```python
from build123d import *

# Parameters (mm, degrees)
BOSS_EXTRUDE1_DEPTH                    = 95
BOSS_EXTRUDE1_DEPTH_BACK               = 105
SKETCH1_R                              = 25
SKETCH2_R                              = 18
BOSS_EXTRUDE2_DEPTH                    = 46
CUT_EXTRUDE1_DEPTH                     = 10
CHAMFER1_SIZE                          = 0.5
SKETCH9_R                              = 10
CUT_EXTRUDE2_DEPTH                     = 30
CUT_EXTRUDE2_DRAFT                     = -8
SKETCH10_R                             = 6.5
CUT_EXTRUDE3_DEPTH                     = 50
SKETCH11_R                             = 6
CUT_EXTRUDE4_DEPTH                     = 249.527664456
CIRPATTERN1_COUNT                      = 4
CUT_EXTRUDE6_START                     = 69
SKETCH21_R                             = 25
SKETCH21_R_2                           = 20
CUT_EXTRUDE6_DEPTH                     = 27
CUT_EXTRUDE7_START                     = -105
SKETCH21_2_R                           = 25
SKETCH21_2_R_2                         = 20
CUT_EXTRUDE7_DEPTH                     = 39
CUT_EXTRUDE8_START                     = -162
SKETCH23_R                             = 25
SKETCH23_R_2                           = 23.75
CUT_EXTRUDE8_DEPTH                     = 135
SKETCH24_R                             = 20
SKETCH24_R_2                           = 19
CUT_EXTRUDE9_DEPTH                     = 20.1
M2_5X0_45_TAPPED_HOLE2_D               = 2.05
M2_5X0_45_TAPPED_HOLE2_DEPTH           = 5
M2_5X0_45_TAPPED_HOLE2_TIP             = 0.615882135
M2_5X0_45_TAPPED_HOLE2_ON_FACE_2_D     = 2.05
M2_5X0_45_TAPPED_HOLE2_ON_FACE_2_DEPTH = 5
M2_5X0_45_TAPPED_HOLE2_ON_FACE_2_TIP   = 0.615882135
CUT_EXTRUDE10_START                    = -12.1
SKETCH25_R                             = 20
SKETCH25_R_2                           = 19
CUT_EXTRUDE10_DEPTH                    = 12.1


with BuildPart() as part:
    # Sketch1 → Boss-Extrude1 (new, two sides: drawn at the far end of the back side and taken through both)
    with BuildSketch(Plane(origin=(0, 0, 0), x_dir=(1, 0, 0), z_dir=(0, 1, 0)).offset(-BOSS_EXTRUDE1_DEPTH_BACK)):
        with Locations(Location((0, 0, 0), (0, 0, 270))):
            Circle(SKETCH1_R)
    extrude(amount=BOSS_EXTRUDE1_DEPTH + BOSS_EXTRUDE1_DEPTH_BACK)

    # Sketch2 → Boss-Extrude2 (add)
    with BuildSketch(Plane(origin=(0, 95, 0), x_dir=(1, 0, 0), z_dir=(0, 1, 0))):
        with Locations(Location((0, 0, 0), (0, 0, 270))):
            Circle(SKETCH2_R)
    extrude(amount=BOSS_EXTRUDE2_DEPTH)

    # Sketch8 → Cut-Extrude1 (cut)
    with BuildSketch(Plane.XY.offset(-15)):
        with BuildLine():
            Line((3, 122), (3, 103))
            ThreePointArc((3, 103), (0, 100), (-3, 103))
            Line((-3, 103), (-3, 122))
            ThreePointArc((-3, 122), (0, 125), (3, 122))
        make_face()
    extrude(amount=-CUT_EXTRUDE1_DEPTH, mode=Mode.SUBTRACT)

    # Chamfer1
    chamfer1_edges = [part.edges().sort_by_distance(p)[0] for p in [
        (0, 141, -18),
    ]]
    chamfer(chamfer1_edges, length=CHAMFER1_SIZE)


with BuildPart() as cut_extrude2_tool:
    # Sketch9 → Cut-Extrude2 (with draft: the straight prism first)
    with BuildSketch(Plane.XZ.offset(105)):
        Circle(SKETCH9_R)
    extrude(amount=-CUT_EXTRUDE2_DEPTH)
    # Cut-Extrude2: the draft: its side faces are tilted about the plane it starts from
    cut_extrude2_sides = [cut_extrude2_tool.faces().sort_by_distance(p)[0] for p in [
        (-10, -90, 0),
    ]]
    draft(cut_extrude2_sides, Plane.XZ.offset(105), CUT_EXTRUDE2_DRAFT)


with BuildPart() as part_1:
    add(part.part)

    # Cut-Extrude2: cut by cut_extrude2_tool
    add(cut_extrude2_tool.part, mode=Mode.SUBTRACT)

    # Sketch10 → Cut-Extrude3 (cut)
    with BuildSketch(Plane.XZ.offset(105)):
        with Locations(Location((0, 0, 0), (0, 0, 270))):
            Circle(SKETCH10_R)
    extrude(amount=-CUT_EXTRUDE3_DEPTH, mode=Mode.SUBTRACT)

    # Sketch11 → Cut-Extrude4 (cut, through all)
    with BuildSketch(Plane(origin=(0, 141, 0), x_dir=(1, 0, 0), z_dir=(0, 1, 0))):
        with Locations(Location((0, 0, 0), (0, 0, 270))):
            Circle(SKETCH11_R)
    extrude(amount=-CUT_EXTRUDE4_DEPTH, mode=Mode.SUBTRACT)

    # Sketch15 → M5x0.8 Tapped Hole1 (revolve, cut)
    with BuildSketch(Plane(origin=(0, 141, -13), x_dir=(0, 0, 1), z_dir=(1, 0, 0))):
        Polygon((0, 0), (0, 12), (2.1, 10.7381927), (2.1, 0), align=None)
    m5x0_8_tapped_hole1 = revolve(axis=Axis((0, 147.35, -13), (0, -1, 0)), mode=Mode.SUBTRACT)

    # CirPattern1: M5x0.8 Tapped Hole1 ×4 about axis
    cirpattern1_axis = Axis((0, 0, 0), (0, 1, 0))
    for i in range(1, CIRPATTERN1_COUNT):
        add(m5x0_8_tapped_hole1.rotate(cirpattern1_axis, i * 360 / CIRPATTERN1_COUNT), mode=Mode.SUBTRACT)

    # Sketch20 → M2.5x0.45 Tapped Hole1 (revolve, cut)
    with BuildSketch(Plane(origin=(12.2, -105, 0), x_dir=(0, 0, -1), z_dir=(1, 0, 0))):
        Polygon((0, 0), (0, 9.35), (1.025, 8.734117865), (1.025, 0), align=None)
    m2_5x0_45_tapped_hole1 = revolve(axis=Axis((12.2, -111.35, 0), (0, 1, 0)), mode=Mode.SUBTRACT)

    # Mirror2: M2.5x0.45 Tapped Hole1 across plane
    add(m2_5x0_45_tapped_hole1.mirror(Plane(origin=(0, 0, 0), x_dir=(0, 0, 1), z_dir=(1, 0, 0))), mode=Mode.SUBTRACT)

    # Sketch21 → Cut-Extrude6 (cut)
    with BuildSketch(Plane(origin=(0, -1, 0), x_dir=(1, 0, 0), z_dir=(0, 1, 0)).offset(CUT_EXTRUDE6_START)):
        with Locations(Location((0, 0, 0), (0, 0, 270))):
            Circle(SKETCH21_R)
        with Locations(Location((0, 0, 0), (0, 0, 270))):
            Circle(SKETCH21_R_2, mode=Mode.SUBTRACT)
    extrude(amount=CUT_EXTRUDE6_DEPTH, mode=Mode.SUBTRACT)

    # Sketch21_2 → Cut-Extrude7 (cut)
    with BuildSketch(Plane(origin=(0, -1, 0), x_dir=(1, 0, 0), z_dir=(0, 1, 0)).offset(CUT_EXTRUDE7_START)):
        with Locations(Location((0, 0, 0), (0, 0, 270))):
            Circle(SKETCH21_2_R)
        with Locations(Location((0, 0, 0), (0, 0, 270))):
            Circle(SKETCH21_2_R_2, mode=Mode.SUBTRACT)
    extrude(amount=CUT_EXTRUDE7_DEPTH, mode=Mode.SUBTRACT)

    # Sketch23 → Cut-Extrude8 (cut)
    with BuildSketch(Plane(origin=(0, 95, 0), x_dir=(1, 0, 0), z_dir=(0, 1, 0)).offset(CUT_EXTRUDE8_START)):
        Circle(SKETCH23_R)
        with Locations(Location((0, 0, 0), (0, 0, 270))):
            Circle(SKETCH23_R_2, mode=Mode.SUBTRACT)
    extrude(amount=CUT_EXTRUDE8_DEPTH, mode=Mode.SUBTRACT)

    # Sketch24 → Cut-Extrude9 (cut)
    with BuildSketch(Plane.XZ.offset(105)):
        with Locations(Location((0, 0, 0), (0, 0, 90))):
            Circle(SKETCH24_R)
        with Locations(Location((0, 0, 0), (0, 0, 270))):
            Circle(SKETCH24_R_2, mode=Mode.SUBTRACT)
    extrude(amount=-CUT_EXTRUDE9_DEPTH, mode=Mode.SUBTRACT)

    # M2.5x0.45 Tapped Hole2
    with Locations(Plane(origin=(0, -99, -19), x_dir=(-1, 0, 0), z_dir=(0, 0, -1))):
        with Locations((0, 0)):
            Hole(M2_5X0_45_TAPPED_HOLE2_D / 2, depth=M2_5X0_45_TAPPED_HOLE2_DEPTH)
            with Locations((0, 0, -(M2_5X0_45_TAPPED_HOLE2_DEPTH + M2_5X0_45_TAPPED_HOLE2_TIP / 2))):  # 118° drill point
                Cone(0, M2_5X0_45_TAPPED_HOLE2_D / 2, M2_5X0_45_TAPPED_HOLE2_TIP, mode=Mode.SUBTRACT)

    # M2.5x0.45 Tapped Hole2 on face 2
    with Locations(Plane(origin=(0, -99, 19), x_dir=(1, 0, 0), z_dir=(0, 0, 1))):
        with Locations((0, 0)):
            Hole(M2_5X0_45_TAPPED_HOLE2_ON_FACE_2_D / 2, depth=M2_5X0_45_TAPPED_HOLE2_ON_FACE_2_DEPTH)
            with Locations((0, 0, -(M2_5X0_45_TAPPED_HOLE2_ON_FACE_2_DEPTH + M2_5X0_45_TAPPED_HOLE2_ON_FACE_2_TIP / 2))):  # 118° drill point
                Cone(0, M2_5X0_45_TAPPED_HOLE2_ON_FACE_2_D / 2, M2_5X0_45_TAPPED_HOLE2_ON_FACE_2_TIP, mode=Mode.SUBTRACT)

    # Sketch25 → Cut-Extrude10 (cut)
    with BuildSketch(Plane(origin=(0, 95, 0), x_dir=(1, 0, 0), z_dir=(0, 1, 0)).offset(CUT_EXTRUDE10_START)):
        with Locations(Location((0, 0, 0), (0, 0, 270))):
            Circle(SKETCH25_R)
        with Locations(Location((0, 0, 0), (0, 0, 90))):
            Circle(SKETCH25_R_2, mode=Mode.SUBTRACT)
    extrude(amount=CUT_EXTRUDE10_DEPTH, mode=Mode.SUBTRACT)


solid = part_1.part
```
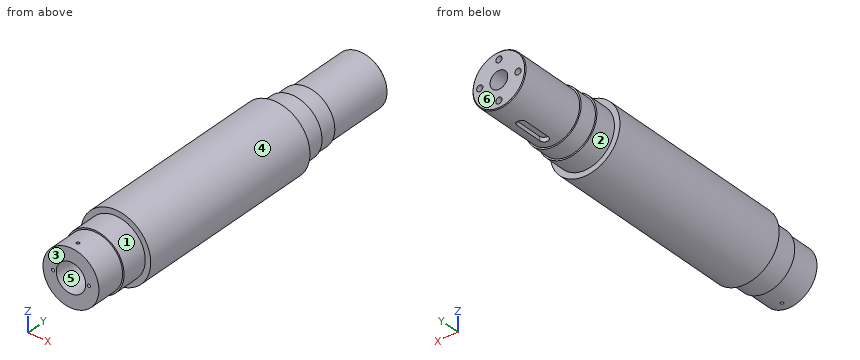
Part model, mm, in its own coordinate system. Face numbers are marked on the shaded views. A direction names the side the tool comes from. Give positions to 0.01 mm unless a question says otherwise; leave off trailing zeros. Order: outer loops, then holes, each group sorted by start corner. A loop starts at its lowest first (then second) coordinate and runs counter-clockwise, first axis right, second up. Notation, with made-up numbers: M 75,42 L 132,42 A34 ccw 132,78 Z; hole C 8,-8 d9. An arc over 180 degrees is marked long. Use a Markdown table: item, result. Add a question column.
(1) Saw through at B-B, the plane y = -31.5. Give the cut face in (x, z), and give its area (3 significant figures).
(2) Drop flat-ended pins along their axis: P1, Ø6.5, axis at x = 0.5, y = 116, coming from the -Z side; P2, Ø2.5, axis at x = 12.2, z = 0, coming from the +Y side; P3, Ø8, axis at y = 108.5, z = -16.5, coming from the +X side. Give the stop position or say it passes through.
(3) Mould opens along X. For the marked faces 4, 5 and 6 say: +X half, -X half, draft (parallel to the pull), parting line (faces both ways), or undercut.
(4) Probe line 1 along X through (y, z) = (-99, 15.35) (3 decimals); line 2 along X through (y, z) = (92.5, 0); line 3 along Y through (x, z) = (0, 16) (3 decimals). List the from-to ranges inside material, lowest first. Write a range as [from, to].
(5) 3-axis set-ups, long thin cutter, end or side, ignore diameter. For the marked faces 1, 2 and 3: which of +Z, -Z, +X, -X, +Y, -Y reach the whole face in a straight line?
(6) Saw through at A-A, the plane y = 114.5. Give the cut face in (x, z).
Answer key:
| question | item | result |
|---|---|---|
| 1 | outline | C 0,0 d47.5; hole C 0,0 d12 |
| 1 | area | 1,660 mm^2 |
| 2 | P1 | z = -17.75 |
| 2 | P2 | y = 130.23 |
| 2 | P3 | x = 12.95 |
| 3 | face 4 | parting line |
| 3 | face 5 | undercut |
| 3 | face 6 | draft |
| 4 | line 1 | [-11.197, -1.025], [1.025, 11.197] |
| 4 | line 2 | [-19, -6], [6, 19] |
| 4 | line 3 | [-105, -100.025], [-97.975, 141] |
| 5 | face 1 | -Y |
| 5 | face 2 | +Y |
| 5 | face 3 | +Z, -Z, +X, -X, -Y |
| 6 | outline | M -3,-17.75 L -3,-15 L 3,-15 L 3,-17.75 A18 ccw long Z; hole C 0,0 d12 |
